Here's the drawing with two shaded views (mm, measured from the low corner). I have some questions. Give positions to 0.01 mm unless a question says otherwise; leave off trailing zeros. Write each loop counter-clockwise with the first axis right and the second up, starting at its lowest first coordinate (ties: lowest second). Pieces come first, ordered by that corner, then holes. Notation, with made-up numbers: (1, -36.75) - (24, -36.75) arc R9 cw to (24, -26.75) - close; hole circle Ø6 at (-25, 22.5). An arc over 180 degrees is marked (long way). Write item = value, one per line.
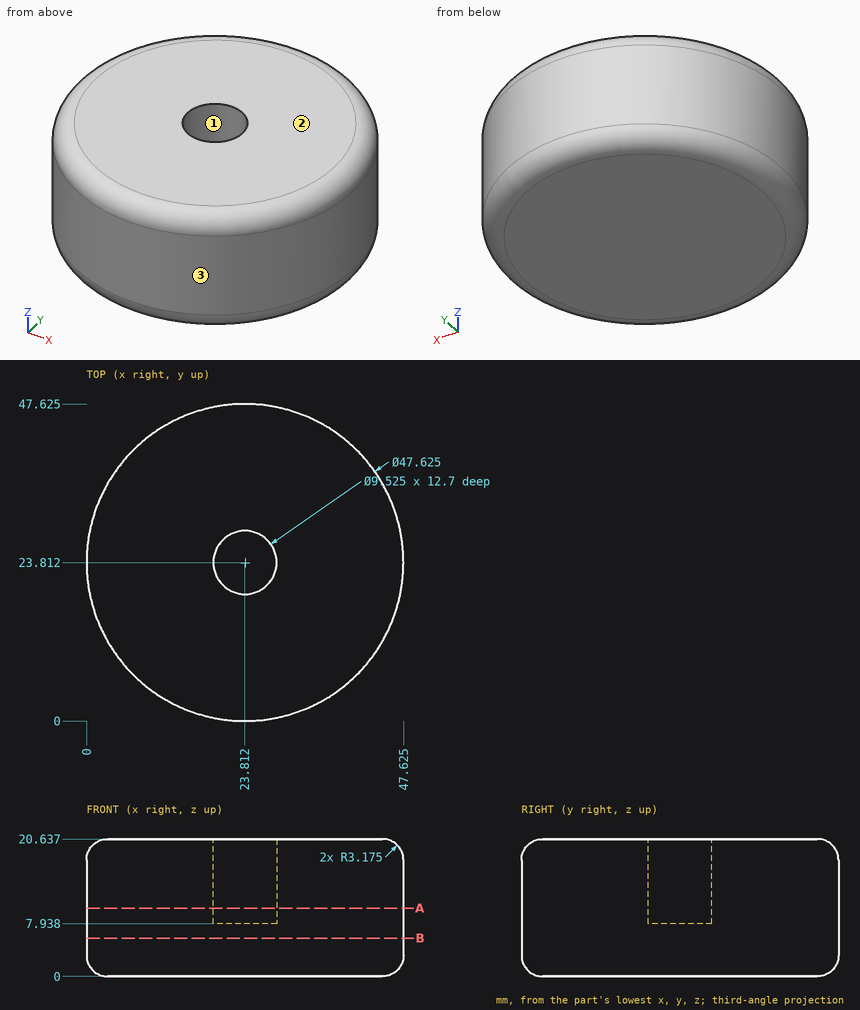
1. Thinking about a two-plate mould opening in Y: for the marked faces 1, 2 and 3, which applies, pulls with the +Y half, pulls with the -Y half, needs draft (parallel to the pull), parting line crosses it, or undercut?
Filled sheet:
face_1 = undercut
face_2 = needs draft
face_3 = parting line crosses it
2. For pin 1 (1 mm diameter, centred on y = 10.5, z = 17, fed in from +X) (1 decimal); pin 2 (2 mm diameter, centred on x = 24.5, y = 31, fed in from -Z); pin 3 (6 mm diameter, centred on x = 24.5, z = 15, fed in from -Y); pin 4 (6 mm diameter, centred on x = 21.5, z = 10.5, fed in from +Y) (1 decimal), each with a flat end and sliding along its axis, tell me the tip position at first contact or that it passes through.
Filled sheet:
pin_1 = 43.9
pin_2 = 0
pin_3 = 0
pin_4 = 47.6
3. I need wall thicknesses on line 1 (Y direction, x = 12, z = 2.75) (1 decimal); line 2 (X direction, y = 27.5, z = 15) (1 decimal); line 3 (X direction, y = 15.5, z = 15). Which ranges of each line are inside material? Lowest first, please.
Filled sheet:
line_1 = 3.2 to 44.5
line_2 = 0.3 to 20.8, 26.8 to 47.3
line_3 = 1.5 to 46.13
4. If we section it at A-A, the plane z = 10.25: Please give me the cut outline in (x, y) (1 decimal).
Filled sheet:
outline = circle Ø47.6 at (23.8, 23.8); hole circle Ø9.5 at (23.8, 23.8)
5. If we section it at B-B, the plane z = 5.75: Please give me the cut outline in (x, y) (1 decimal).
Filled sheet:
outline = circle Ø47.6 at (23.8, 23.8)
